Geometry: final body of the model. Coordinates: model frame, mm. A direction names the side the tool comes from. Give positions to 0.01 mm unless a question says otherwise; leave off trailing zeros. Loops run counter-clockwise (first coordinate to the right, second up) from the corner with the lowest first, then second, coordinate; pieces in that order, holes last. Notation, with made-up numbers: (16.25, 42) - (63.25, 42) arc R36 cw to (63.25, 81) - close; hole circle Ø7 at (37, 66.25). An arc over 180 degrees is marked (long way). Answer in a Markdown table with one row per item.
from build123d import *

# Parameters (mm, degrees)
SKETCH_W     = 50
SKETCH_H     = 50
SKETCH_R     = 11
PAD_DEPTH    = 5
SKETCH001_W  = 50
SKETCH001_H  = 50
SKETCH001_R  = 5.5
PAD001_DEPTH = 1


with BuildPart() as part:
    # Sketch → Pad (new body)
    with BuildSketch(Plane.XY):
        with Locations((25, 25)):
            Rectangle(SKETCH_W, SKETCH_H)
        with Locations((25, 25)):
            Circle(SKETCH_R, mode=Mode.SUBTRACT)
    extrude(amount=PAD_DEPTH)

    # Sketch001 → Pad001 (new body)
    with BuildSketch(Plane.XY.offset(5)):
        with Locations((25, 25)):
            Rectangle(SKETCH001_W, SKETCH001_H)
        with Locations((25, 25)):
            Circle(SKETCH001_R, mode=Mode.SUBTRACT)
    extrude(amount=PAD001_DEPTH)


solid = part.part
Q1. Reachability of faces 1 (the flat face through (22, 30, 5)), 2 (the flat face through (0, 25, 3)) from +Z, -Z, +X, -X, +Y, -Y: full face, straight path, thin tool, end or side. Return the list, or none.
Check values:
| item | result |
|---|---|
| face 1 | -Z |
| face 2 | +Z, -Z, -X, +Y, -Y |
Q2. First-contact query: pin 1 (17.5 mm diameter, centred on x = 25, y = 25, fed in from -Z). Flat tip, straight axial feed; report the tip coordinate or a pass-through.
Check values:
| item | result |
|---|---|
| pin 1 | z = 5 |
Q3. Cut plane A-A (x = 25). Output: boundary loops of the cut face in (y, z), and give its area (3 significant figures).
Check values:
| item | result |
|---|---|
| outline | (0, 0) - (14, 0) - (14, 5) - (19.5, 5) - (19.5, 6) - (0, 6) - close; (30.5, 5) - (36, 5) - (36, 0) - (50, 0) - (50, 6) - (30.5, 6) - close |
| area | 179 mm² |
Q4. Material intervals for line 1 along Y through (x, z) = (25, 5.6); line 2 along Y through (x, z) = (25, 3.4); line 3 along X through (y, z) = (17, 0.7), sorted ascending.
Check values:
| item | result |
|---|---|
| line 1 | 0 to 19.5, 30.5 to 50 |
| line 2 | 0 to 14, 36 to 50 |
| line 3 | 0 to 17.45, 32.55 to 50 |
Q5. Cut plane C-C (z = 4.2). Output: boundary loops of the cut face in (x, y), and give its area (3 significant figures).
Check values:
| item | result |
|---|---|
| outline | (0, 0) - (50, 0) - (50, 50) - (0, 50) - close; hole circle Ø22 at (25, 25) |
| area | 2,120 mm² |
Q6. Cut plane D-D (x = 15). Output: boundary loops of the cut face in (y, z).
Check values:
| item | result |
|---|---|
| outline | (0, 0) - (20.42, 0) - (20.42, 5) - (29.58, 5) - (29.58, 0) - (50, 0) - (50, 6) - (0, 6) - close |
Q7. Draft query along X for faces 3 (the cylindrical face through (35.161, 20.787, 2.465)), 4 (the flat face through (19, 25, 6)), 5 (the flat face through (50, 25, 3)). Return one class per face: pulls with the +X half, pulls with the -X half, needs draft (parallel to the pull), parting line crosses it, or undercut.
Check values:
| item | result |
|---|---|
| face 3 | undercut |
| face 4 | needs draft |
| face 5 | pulls with the +X half |
